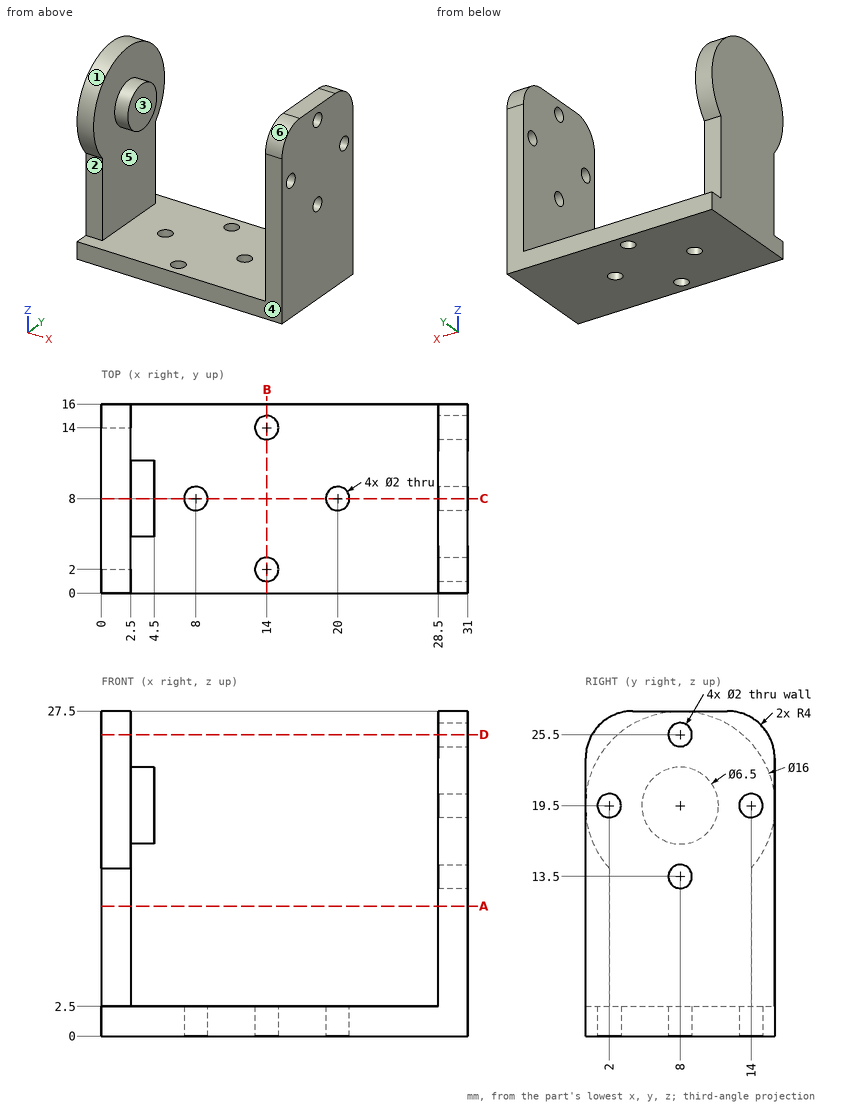
Part print with two shaded views. Sizes in mm from the minimum x, y, z corner. A direction names the side the tool comes from. Round coordinates to 2 decimals unless told otherwise and drop trailing zeros. Write each loop counter-clockwise with the first axis right and the second up, starting at its lowest first coordinate (ties: lowest second). Pieces come first, ordered by that corner, then holes. Notation, with made-up numbers: M 33,-20 L 86,-20 A17 ccw 86,-3 Z; hole C -32,32 d1. An arc over 180 degrees is marked long. Put each result on its own line as item: value. Start each with the question number.
1) Pull direction Z, two halves, no side cores. Call the marked faces 4, 5 and 6: pulls with the +Z half, pulls with the -Z half, needs draft (parallel to the pull), parting line crosses it, or undercut.
2) Saw through at B-B, the plane x = 14. Write the cut outline in (y, z).
3) Drill centre lines: probe 1 along Y at (x, z) = (14, 1.55); probe 2 along X at (y, z) = (6, 22.75); probe 3 along Z at (x, y) = (3.5, 11.75). Where is each one in solid material? Low to high. Write a range as [from, to].
4) Saw through at D-D, the plane z = 25.5. Write the cut outline in (x, y).
5) Saw through at A-A, the plane z = 11. Write the cut outline in (x, y), and give its area (3 significant figures).
6) 3-axis set-ups, long thin cutter, end or side, ignore diameter. For the marked faces 1, 2 and 3: which of +Z, -Z, +X, -X, +Y, -Y reach the whole face in a straight line?
7) Pin check, flat tips, straight feed: pin 1 Ø4 at (x, y) = (25, 7.5) entering from +Z; pin 2 Ø1.2 at (x, z) = (1, 9) entering from +Y; pin 3 Ø0.8 at (x, z) = (1.5, 11.5) entering from -Y. Stop position of each tip, or through.
8) Saw through at C-C, the plane y = 8. Write the cut outline in (x, z), and give its area (4 significant figures).
Resolved:
1. face 4: needs draft
1. face 5: undercut
1. face 6: pulls with the +Z half
2. outline: M 0,0 L 1,0 L 1,2.5 L 0,2.5 Z; M 3,0 L 13,0 L 13,2.5 L 3,2.5 Z; M 15,0 L 16,0 L 16,2.5 L 15,2.5 Z
3. probe 1: [0, 1], [3, 13], [15, 16]
3. probe 2: [0, 2.5], [28.5, 31]
3. probe 3: [0, 2.5]
4. outline: M 0,2.71 L 2.5,2.71 L 2.5,13.29 L 0,13.29 Z; M 28.5,0.54 L 31,0.54 L 31,7 L 28.5,7 Z; M 28.5,9 L 31,9 L 31,15.46 L 28.5,15.46 Z
5. outline: M 0,2 L 2.5,2 L 2.5,14 L 0,14 Z; M 28.5,0 L 31,0 L 31,16 L 28.5,16 Z
5. area: 70.0 mm²
6. face 1: -X
6. face 2: -X, -Y
6. face 3: +Z, +Y, -Y
7. pin 1: z = 2.5
7. pin 2: y = 14
7. pin 3: y = 2
8. outline: M 0,0 L 7,0 L 7,2.5 L 2.5,2.5 L 2.5,16.25 L 4.5,16.25 L 4.5,22.75 L 2.5,22.75 L 2.5,27.5 L 0,27.5 Z; M 9,0 L 19,0 L 19,2.5 L 9,2.5 Z; M 21,0 L 31,0 L 31,12.5 L 28.5,12.5 L 28.5,2.5 L 21,2.5 Z; M 28.5,14.5 L 31,14.5 L 31,24.5 L 28.5,24.5 Z; M 28.5,26.5 L 31,26.5 L 31,27.5 L 28.5,27.5 Z
8. area: 195.5 mm²
